Work out the finished part from the listing and answer in its coordinate system (mm). A direction names the side the tool comes from. Coordinates: 2 decimals unless noted, no trailing zeros. Order: outer loops, then holes, each group sorted by start corner. A loop starts at its lowest first (then second) coordinate and runs counter-clockwise, first axis right, second up. Notation, with made-up numbers: M 2,29 L 46,29 A10 cw 46,44 Z; hole C -31.75,0 d4. An arc over 180 degrees is marked long. Use a Markdown table: item, result. Add a question column.
from build123d import *

# Parameters (mm, degrees)
SKETCH1_R           = 12.5381004
BOSS_EXTRUDE1_DEPTH = 47
SKETCH2_W           = 88.9
SKETCH2_H           = 47
BOSS_EXTRUDE2_DEPTH = 6.35
FILLET1_R           = 6.35
SKETCH3_R           = 1.5875
CUT_EXTRUDE1_DEPTH  = 9.525
BOSS_EXTRUDE3_START = 4.7625
SKETCH5_R           = 3.5381057
SKETCH5_R_2         = 1.538097
BOSS_EXTRUDE3_DEPTH = 4.7625


with BuildPart() as part:
    # Sketch1 → Boss-Extrude1 (new body)
    with BuildSketch(Plane.XY):
        with BuildLine():
            Line((-25.4, 22.225), (25.4, 22.225))
            Line((25.4, 22.225), (21.680256121, -3.175))
            ThreePointArc((21.680256121, -3.175), (0, -21.911506805), (-21.680256121, -3.175))
            Line((-21.680256121, -3.175), (-25.4, 22.225))
        make_face()
        Circle(SKETCH1_R, mode=Mode.SUBTRACT)
    extrude(amount=-BOSS_EXTRUDE1_DEPTH)

    # Sketch2 → Boss-Extrude2 (add)
    with BuildSketch(Plane(origin=(0, 22.225, 0), x_dir=(1, 0, 0), z_dir=(0, 1, 0))):
        with Locations((0, 23.5)):
            Rectangle(SKETCH2_W, SKETCH2_H)
    extrude(amount=-BOSS_EXTRUDE2_DEPTH)

    # Fillet1
    fillet1_edges = [part.edges().sort_by_distance(p)[0] for p in [
        (44.45, 15.875, -23.5),
        (-44.45, 15.875, -23.5),
        (24.47006403, 15.875, -23.5),
        (-24.47006403, 15.875, -23.5),
    ]]
    fillet(fillet1_edges, radius=FILLET1_R - 0.0001)  # a hair under: the kernel refuses the full size

    # Sketch3 → Cut-Extrude1 (cut)
    with BuildSketch(Plane.XZ.offset(-15.875)):
        with Locations(Location((-34.036, -7.625, 0), (0, 0, 270))):
            Circle(SKETCH3_R)
        with Locations(Location((-34.036, -39.375, 0), (0, 0, 270))):
            Circle(SKETCH3_R)
        with Locations(Location((34.036, -39.375, 0), (0, 0, 270))):
            Circle(SKETCH3_R)
        with Locations(Location((34.036, -7.625, 0), (0, 0, 270))):
            Circle(SKETCH3_R)
    extrude(amount=-CUT_EXTRUDE1_DEPTH, mode=Mode.SUBTRACT)

    # Sketch5 → Boss-Extrude3 (add)
    with BuildSketch(Plane.XY.offset(BOSS_EXTRUDE3_START)):
        with BuildLine():
            Line((29.957859818, 15.875), (38.1, 15.875))
            ThreePointArc((38.1, 15.875), (42.590128061, 17.734871939), (44.45, 22.225))
            Line((44.45, 22.225), (-44.45, 22.225))
            ThreePointArc((-44.45, 22.225), (-42.590128061, 17.734871939), (-38.1, 15.875))
            Line((-38.1, 15.875), (-29.957859818, 15.875))
            ThreePointArc((-29.957859818, 15.875), (-25.805768294, 14.329439195), (-23.674876744, 10.445121568))
            Line((-23.674876744, 10.445121568), (-21.680256121, -3.175))
            ThreePointArc((-21.680256121, -3.175), (0, -21.911506805), (21.680256121, -3.175))
            Line((21.680256121, -3.175), (23.674876744, 10.445121568))
            ThreePointArc((23.674876744, 10.445121568), (25.805768294, 14.329439195), (29.957859818, 15.875))
        make_face()
        with Locations(Location((0, 0, 0), (0, 0, 180))):
            Circle(SKETCH5_R, mode=Mode.SUBTRACT)
        with Locations(Location((-8.5, 0, 0), (0, 0, 180))):
            Circle(SKETCH5_R_2, mode=Mode.SUBTRACT)
        with Locations(Location((8.5, 0, 0), (0, 0, 180))):
            Circle(SKETCH5_R_2, mode=Mode.SUBTRACT)
    extrude(amount=-BOSS_EXTRUDE3_DEPTH)


solid = part.part
(1) The mould has two halves that part along X. Classify faces 3 (the cylindrical face through (-6.963, -0.068, 2.415)), 4 (the cylindrical face through (25.76, 14.29, 2.41)), 5 (the flat face through (34, 15.875, -21)): pulls with the +X half, pulls with the -X half, needs draft (parallel to the pull), parting line crosses it, or undercut.
(2) A cutting plane is placed at A-A on x = 0. Write down the section's boundary in (y, z) (1 decimal).
(3) Straight lines are drawn through the part: line 1 (Y direction, x = 0, z = -15.5) (1 decimal); line 2 (Y direction, x = 0, z = 2.25) (1 decimal); line 3 (X direction, y = -10, z = -26.5). For each, find the intervals that lie inside material, in ascending order.
(4) Given P1, Ø9, axis at x = 35.5, z = -32, coming from the -Y side (3 decimals); P2, Ø11.5, axis at x = 0, y = 0, coming from the -Z side; P3, Ø5, axis at x = 19.5, z = -16.5, coming from the -Y side, each flat-ended and moving along its own axis, determine where each tip first touches the part or whether it passes through.
(5) Which of the six approach directions +Z, -Z, +X, -X, +Y, -Y give full straight-line access (tool end or side, diameter ignored) to faces 1 (the cylindrical face through (-2.72, -12.24, -23.17)), 2 (the cylindrical face through (-34.644, 19.006, -9.091))?
(6) A cutting plane is placed at C-C on y = 20. Count the separate pieces of the cut face and the enclosed holes in it, plus the area to 3 significant figures.
From the geometry:
| question | item | result |
|---|---|---|
| 1 | face 3 | undercut |
| 1 | face 4 | pulls with the +X half |
| 1 | face 5 | needs draft |
| 2 | outline | M -21.9,-47 L -12.5,-47 L -12.5,0 L -3.5,0 L -3.5,4.8 L -21.9,4.8 Z; M 3.5,0 L 12.5,0 L 12.5,-47 L 22.2,-47 L 22.2,4.8 L 3.5,4.8 Z |
| 3 | line 1 | y = -21.9 to -12.5, 12.5 to 22.2 |
| 3 | line 2 | y = -21.9 to -3.5, 3.5 to 22.2 |
| 3 | line 3 | x = -19.5 to -7.56, 7.56 to 19.5 |
| 4 | P1 | stops at y = 15.875 |
| 4 | P2 | stops at z = 0 |
| 4 | P3 | stops at y = -13.82 |
| 5 | face 1 | -Z |
| 5 | face 2 | +Y, -Y |
| 6 | separate pieces | 1 |
| 6 | enclosed holes | 4 |
| 6 | area | 4,530 mm2 |
